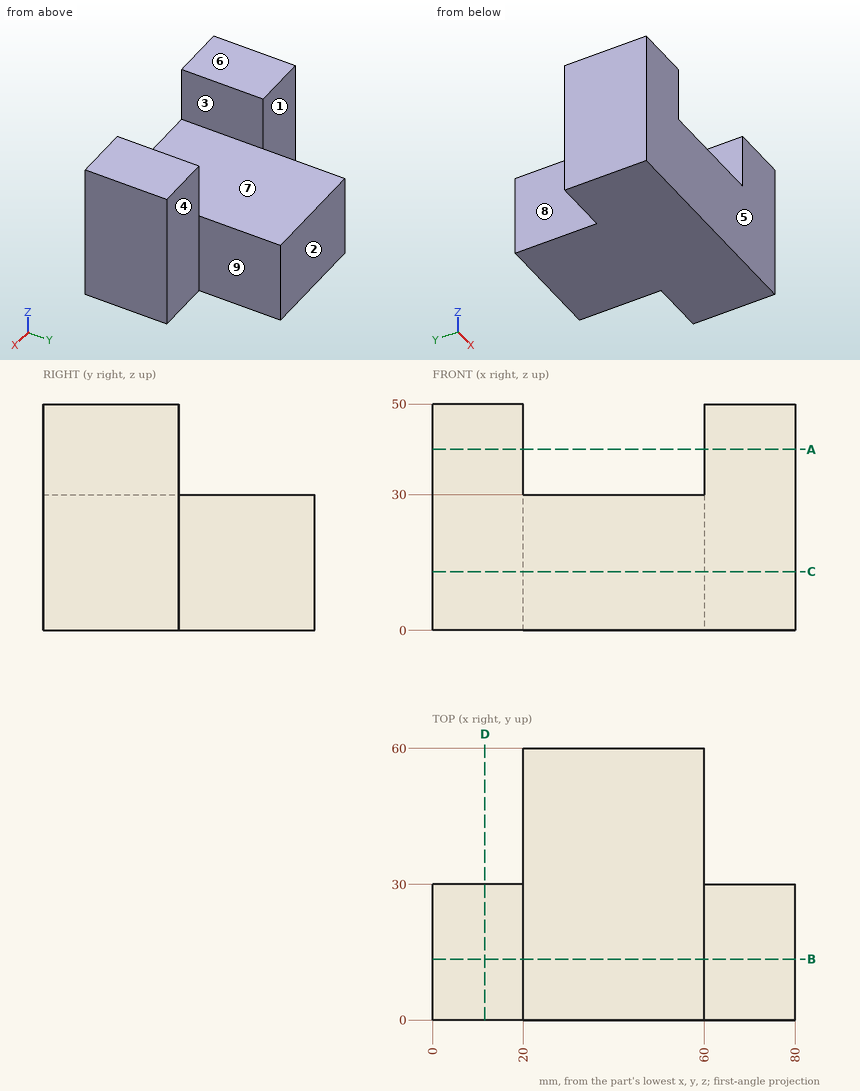
Part print with two shaded views. Sizes in mm from the minimum x, y, z corner. A direction names the side the tool comes from. Round coordinates to 2 decimals unless told otherwise and drop trailing zeros. Order: outer loops, then holes, each group sorted by start corner. A loop starts at its lowest first (then second) coordinate and runs counter-clockwise, first axis right, second up. Notation, with made-up numbers: M -12,74 L -8,74 A13 ccw -8,90 Z; hole C 47,20.25 d10. An arc over 180 degrees is marked long. Answer in a Markdown table with one row per item. Add a question column.
Q1. Pin check, flat tips, straight feed: pin 1 (20 mm diameter, centred on x = 35, y = 42, fed in from +Z); pin 2 (24 mm diameter, centred on y = 51.5, z = 13.5, fed in from -X); pin 3 (15 mm diameter, centred on y = 47, z = 9, fed in from +X); pin 4 (8 mm diameter, centred on y = 44.5, z = 36.5, fed in from -X). Stop position of each tip, or through.
Q2. Cut at A-A on z = 40. Give the cut face in (x, y).
Q3. Cut at C-C on z = 13. Give the cut face in (x, y), and give its area (3 significant figures).
Q4. Cut at D-D on x = 11.5. Give the cut face in (y, z), and give its area (3 significant figures).
Q5. Mould opens along X. For the marked faces 6, 7, 8 and 9 say: +X half, -X half, draft (parallel to the pull), parting line (faces both ways), or undercut.
Q6. Cut at B-B on y = 13.5. Give the cut face in (x, z).
Q7. 3-axis set-ups, long thin cutter, end or side, ignore diameter. For the marked faces 1, 2, 3, 4 and 5: which of +Z, -Z, +X, -X, +Y, -Y reach the whole face in a straight line?
Q8. Wall check: L1, parallel to X at y = 16, z = 39.5; L2, parallel to X at y = 40.5, z = 24; L3, parallel to Z at x = 37, y = 8.5. Give the ranges that are in metal, low to high. Write a range as from..to.
Established:
| question | item | result |
|---|---|---|
| 1 | pin 1 | stops at z = 30 |
| 1 | pin 2 | stops at x = 20 |
| 1 | pin 3 | stops at x = 60 |
| 1 | pin 4 | passes through |
| 2 | outline | M 0,0 L 20,0 L 20,30 L 0,30 Z; M 60,0 L 80,0 L 80,30 L 60,30 Z |
| 3 | outline | M 0,0 L 80,0 L 80,30 L 60,30 L 60,60 L 20,60 L 20,30 L 0,30 Z |
| 3 | area | 3,600 mm2 |
| 4 | outline | M 0,0 L 30,0 L 30,50 L 0,50 Z |
| 4 | area | 1,500 mm2 |
| 5 | face 6 | draft |
| 5 | face 7 | undercut |
| 5 | face 8 | -X half |
| 5 | face 9 | +X half |
| 6 | outline | M 0,0 L 80,0 L 80,50 L 60,50 L 60,30 L 20,30 L 20,50 L 0,50 Z |
| 7 | face 1 | +Z, -Z, -X, +Y |
| 7 | face 2 | +Z, -Z, +X, -X, +Y |
| 7 | face 3 | +Z, +Y, -Y |
| 7 | face 4 | +Z, -Z, +X, +Y |
| 7 | face 5 | +Z, -Z, +X, -X, -Y |
| 8 | L1 | x = 0..20, 60..80 |
| 8 | L2 | x = 20..60 |
| 8 | L3 | z = 0..30 |
